Autodesk Inventor part; units mm, degrees
ref_plane "YZ Plane" through (0, 0, 0) normal (1, 0, 0) x (0, 1, 0)
ref_plane "XZ Plane" through (0, 0, 0) normal (0, 1, 0) x (-1, 0, 0)
ref_plane "XY Plane" through (0, 0, 0) normal (0, 0, 1) x (1, 0, 0)
sketch "Sketch1" plane through (0, 0, 0) normal (0, 0, 1) x (1, 0, 0)
  line L0 (0, 0) -> (220, 0)
  line L1 (220, 0) -> (220, 60)
  line L2 (220, 60) -> (0, 60)
  line L3 (0, 60) -> (0, 0)
  dimension "d0" = 220
  dimension "d1" = 60
extrude "Extrusion1" add sketch "Sketch1" along normal blind 3
sketch "Sketch2" plane through (0, 0, 3) normal (0, 0, 1) x (1, 0, 0)
  line L0 (0, 60) -> (0, 0)
  line L1 (0, 0) -> (0, 3)
  line L2 (0, 0) -> (3, 0) construction
  line L3 (0, 3) -> (220, 3)
  line L4 (220, 3) -> (220, 6)
  line L5 (220, 6) -> (0, 6)
  line L6 (0, 6) -> (0, 3)
  dimension "d4" = 3
  dimension "d5" = 90
  dimension "d6" = 220
  dimension "d7" = 3
extrude "Extrusion2" cut sketch "Sketch2" against normal blind 1.5
chamfer "Chamfer1" distance 3 angle 45 1 edges at (0, 33, 3)
chamfer "Chamfer2" distance 3 angle 45 1 edges at (220, 33, 3)
properties part number "Inert sider"
Design review of the part built by this model. Coordinates are the model's own, in mm. Give positions to 0.01 mm unless a question says otherwise; leave off trailing zeros. Write each loop counter-clockwise with the first axis right and the second up, starting at its lowest first coordinate (ties: lowest second). Pieces come first, ordered by that corner, then holes. Notation, with made-up numbers: (10, 73) -> (17, 73) arc R23 ccw to (17, 93) -> close; hole circle Ø8 at (51.5, 31). An arc over 180 degrees is marked (long way). Answer in a Markdown table with one row per item.
(1) Consider section B-B (x = 24). State the section outline as (y, z) points.
Results:
| item | result |
|---|---|
| outline | (0, 0) -> (60, 0) -> (60, 3) -> (6, 3) -> (6, 1.5) -> (3, 1.5) -> (3, 3) -> (0, 3) -> close |
(2) Clearance check with flat-ended pins moving along their axes: pin 1 (1.5 mm diameter, centred on y = 11, z = 1.5, fed in from -X); pin 2 (3.5 mm diameter, centred on x = 142.5, y = 4.5, fed in from +Z). State where each tip first meets the part, or that it passes through.
Results:
| item | result |
|---|---|
| pin 1 | x = 0.75 |
| pin 2 | z = 3 |
(3) Consider section A-A (z = 2). State the section outline as (x, y) points, then the cut area to 3 significant figures.
Results:
| item | result |
|---|---|
| outline | (2, 0) -> (218, 0) -> (218, 3) -> (2, 3) -> close; (2, 6) -> (218, 6) -> (218, 60) -> (2, 60) -> close |
| area | 12,300 mm2 |
(4) To check wall thickness, follow probe 1 along Y at (x, z) = (198, 1.7); probe 2 along X at (y, z) = (50.5, 0.75); probe 3 along X at (y, z) = (24.5, 0.2). State the ranges of each line that lie inside material, in increasing order.
Results:
| item | result |
|---|---|
| probe 1 | 0 to 3, 6 to 60 |
| probe 2 | 0.75 to 219.25 |
| probe 3 | 0.2 to 219.8 |
